For this review, take the finished solid that the model builds, in its own axes (mm). A direction names the side the tool comes from. Coordinates: 2 decimals unless noted, no trailing zeros. Order: outer loops, then holes, each group sorted by start corner. A loop starts at its lowest first (then second) coordinate and runs counter-clockwise, first axis right, second up. Notation, with made-up numbers: (50, 78) -> (108, 78) arc R23 ccw to (108, 110) -> close; hole circle Ø3 at (72.5, 48.25). An arc over 180 degrees is marked (long way). Write item = value, one per line. Start each with the question number.
1) Machinability: for faces 1 (the face through (-18, 6.5, 1)), 2 (the face through (-24, 8, 6)), 3 (the face through (-4, 8, 10)), 4 (the face through (-148, 10, 10)), which of the approach directions +Z, -Z, +X, -X, +Y, -Y give a long, thin tool a straight path to every point of the face, cutting with its end or side? Answer none if there is none.
2) Insertion check: pin 1 Ø4.5 at (x, y) = (-105, 8) entering from -Z; pin 2 Ø1.2 at (x, y) = (-198, 8.5) entering from +Z. Each pin has a flat end and moves straight along its axis. Give the tip position at first contact, or say it passes through.
3) Consider section A-A on x = -105. Give the boundary of the cut face in (y, z), and give its area (3 significant figures).
4) Consider section D-D on x = -157.5. Give the boundary of the cut face in (y, z).
5) Consider section C-C on z = 5.25. Give the boundary of the cut face in (x, y), and give its area (3 significant figures).
6) Consider section B-B on y = 8. State how many separate pieces and enclosed holes the cut face has, and give its area (3 significant figures).
7) Wall thickness on probe 1 along Y at (x, z) = (-150, 11); probe 2 along X at (y, z) = (8, 5.5); probe 3 along X at (y, z) = (9.5, 3): over which ranges is each line inside the solid? List them lowest first. Write a range as [from, to].
8) Draft analysis for pull direction Y (two halves, no side actions). For faces 5 (the face through (-7, 13, 10)), 6 (the face through (-9, 8, 7)), state which applies: +Y half, -Y half, draft (parallel to the pull), parting line (faces both ways), or undercut.
from build123d import *

# Parameters (mm, degrees)
F0_W     = 200
F0_H     = 16
F1_DEPTH = 12
F2_W     = 196
F2_H     = 4
F3_DEPTH = 5
F4_R     = 4
F5_DEPTH = 10
F7_D     = 5
F8_W     = 3
F8_H     = 6
F9_DEPTH = 5


with BuildPart() as f1:
    # F0 (on Top) → F1 (new body)
    with BuildSketch(Plane.XY):
        with Locations((-100, 8)):
            Rectangle(F0_W, F0_H)
    extrude(amount=F1_DEPTH)

    # F2 (on face) → F3 (cut)
    with BuildSketch(Plane.XY.offset(12)):
        with Locations((-102, 8)):
            Rectangle(F2_W, F2_H)
    extrude(amount=-F3_DEPTH, mode=Mode.SUBTRACT)

    # F4 (on face) → F5 (cut)
    with BuildSketch(Plane.XY.offset(12)):
        with Locations((-190, 8)):
            Circle(F4_R)
        with Locations((-105, 8)):
            Circle(F4_R)
        with Locations((-20, 8)):
            Circle(F4_R)
    extrude(amount=-F5_DEPTH, mode=Mode.SUBTRACT)

    # F7 (through all)
    with Locations(Plane.XY.offset(12)):
        with Locations((-105, 8), (-190, 8), (-20, 8)):
            Hole(F7_D / 2)

    # F8 (on face) → F9 (cut)
    with BuildSketch(Plane.XY.offset(12)):
        with Locations((-5.5, 13)):
            Rectangle(F8_W, F8_H)
        with Locations((-5.5, 3)):
            Rectangle(F8_W, F8_H)
    extrude(amount=-F9_DEPTH, mode=Mode.SUBTRACT)


solid = f1.part
Answer sheet:
q1.face_1 = +Z, -Z
q1.face_2 = +Z
q1.face_3 = +Z, +Y, -Y
q1.face_4 = +Z, -X
q2.pin_1 = through
q2.pin_2 = 7
q3.outline = (0, 0) -> (5.5, 0) -> (5.5, 2) -> (4, 2) -> (4, 12) -> (0, 12) -> close; (10.5, 0) -> (16, 0) -> (16, 12) -> (12, 12) -> (12, 2) -> (10.5, 2) -> close
q3.area = 102 mm2
q4.outline = (0, 0) -> (16, 0) -> (16, 12) -> (10, 12) -> (10, 7) -> (6, 7) -> (6, 12) -> (0, 12) -> close
q5.outline = (-200, 0) -> (0, 0) -> (0, 16) -> (-200, 16) -> close; hole circle Ø8 at (-190, 8); hole circle Ø8 at (-105, 8); hole circle Ø8 at (-20, 8)
q5.area = 3,050 mm2
q6.separate_pieces = 4
q6.enclosed_holes = 0
q6.area = 1,270 mm2
q7.probe_1 = [0, 6], [10, 16]
q7.probe_2 = [-200, -194], [-186, -109], [-101, -24], [-16, 0]
q7.probe_3 = [-200, -193.71], [-186.29, -108.71], [-101.29, -23.71], [-16.29, 0]
q8.face_5 = draft
q8.face_6 = undercut
